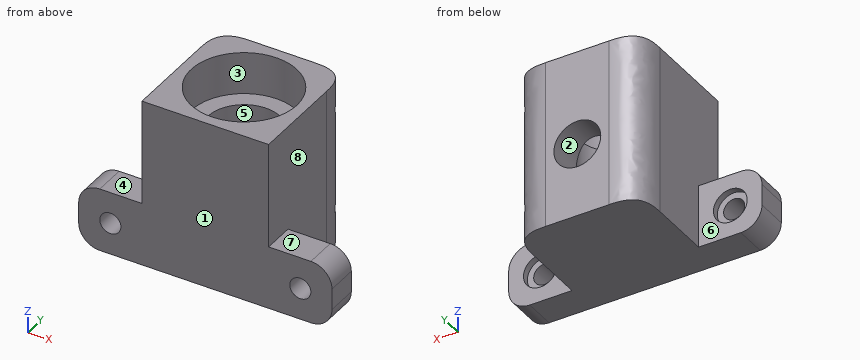
from build123d import *

# Parameters (mm, degrees)
BOSS_EXTRUDE1_DEPTH      = 35
BOSS_EXTRUDE1_DEPTH_BACK = 5
SKETCH1_W                = 30
SKETCH1_H                = 30
FILLET1_SIZE             = 7.5
SKETCH2_R                = 8.5
CUT_EXTRUDE1_DEPTH       = 60
SKETCH3_W                = 15
SKETCH3_H                = 7.5
BOSS_EXTRUDE2_DEPTH      = 15
SKETCH5_W                = 15
SKETCH5_H                = 7.5
BOSS_EXTRUDE4_DEPTH      = 15
SKETCH11_R               = 12.5
CUT_EXTRUDE3_DEPTH       = 10
FILLET8_R                = 5
SKETCH15_R               = 4
CUT_EXTRUDE5_DEPTH       = 1.5
SKETCH19_R               = 5.55625
CUT_EXTRUDE10_DEPTH      = 11.5
SKETCH21_R               = 2.5
CUT_EXTRUDE11_DEPTH      = 11.5


with BuildPart() as part:
    # Sketch1 → Boss-Extrude1 (new, two sides: drawn at the far end of the back side and taken through both)
    with BuildSketch(Plane.XY.offset(-BOSS_EXTRUDE1_DEPTH_BACK)):
        Rectangle(SKETCH1_W, SKETCH1_H)
    extrude(amount=BOSS_EXTRUDE1_DEPTH + BOSS_EXTRUDE1_DEPTH_BACK)

    # Fillet1
    # a fillet whose section is not a circle: 7.5 mm, written as the material it takes off along each edge
    with BuildSketch(Plane(origin=(-15, 15, 53.75), x_dir=(1, 0, 0), z_dir=(0, 0, -1))) as fillet1_piece_1:
        with BuildLine():
            add(Edge.make_bspline([(FILLET1_SIZE, 0), (FILLET1_SIZE * 0.831801948466, 0), (FILLET1_SIZE * 0.663603896932, 0), (FILLET1_SIZE * 0.292893218813, FILLET1_SIZE * 0.0716919198361), (FILLET1_SIZE * 0.0716919198361, FILLET1_SIZE * 0.292893218813), (0, FILLET1_SIZE * 0.663603896932), (0, FILLET1_SIZE * 0.831801948466), (0, FILLET1_SIZE)], knots=[0, 0, 0, 0, 0, 0, 0.5, 0.5, 1, 1, 1, 1, 1, 1], degree=5))
            Line((0, FILLET1_SIZE), (0, 0))
            Line((0, 0), (FILLET1_SIZE, 0))
        make_face()
    extrude(amount=77.5, mode=Mode.SUBTRACT)
    with BuildSketch(Plane(origin=(15, 15, -23.75), x_dir=(0, -1, 0), z_dir=(0, 0, 1))) as fillet1_piece_2:
        with BuildLine():
            add(Edge.make_bspline([(FILLET1_SIZE, 0), (FILLET1_SIZE * 0.831801948466, 0), (FILLET1_SIZE * 0.663603896932, 0), (FILLET1_SIZE * 0.292893218813, -FILLET1_SIZE * 0.0716919198361), (FILLET1_SIZE * 0.0716919198361, -FILLET1_SIZE * 0.292893218813), (0, -FILLET1_SIZE * 0.663603896932), (0, -FILLET1_SIZE * 0.831801948466), (0, -FILLET1_SIZE)], knots=[0, 0, 0, 0, 0, 0, 0.5, 0.5, 1, 1, 1, 1, 1, 1], degree=5))
            Line((0, -FILLET1_SIZE), (0, 0))
            Line((0, 0), (FILLET1_SIZE, 0))
        make_face()
    extrude(amount=77.5, mode=Mode.SUBTRACT)

    # Sketch2 → Cut-Extrude1 (cut)
    with BuildSketch(Plane.XY):
        with Locations(Location((0, 0, 0), (0, 0, 180))):
            Circle(SKETCH2_R)
    extrude(amount=CUT_EXTRUDE1_DEPTH, mode=Mode.SUBTRACT)

    # Sketch3 → Boss-Extrude2 (add)
    with BuildSketch(Plane(origin=(15, 0, 0), x_dir=(0, 0, -1), z_dir=(1, 0, 0))):
        with Locations((-2.5, -11.25)):
            Rectangle(SKETCH3_W, SKETCH3_H)
    extrude(amount=BOSS_EXTRUDE2_DEPTH)

    # Sketch5 → Boss-Extrude4 (add)
    with BuildSketch(Plane.ZY.offset(15)):
        with Locations((2.5, -11.25)):
            Rectangle(SKETCH5_W, SKETCH5_H)
    extrude(amount=BOSS_EXTRUDE4_DEPTH)

    # Sketch11 → Cut-Extrude3 (cut)
    with BuildSketch(Plane.XY.offset(35)):
        Circle(SKETCH11_R)
    extrude(amount=-CUT_EXTRUDE3_DEPTH, mode=Mode.SUBTRACT)

    # Fillet8
    fillet8_edges = [part.edges().sort_by_distance(p)[0] for p in [
        (30, -11.25, -5),
        (30, -11.25, 10),
        (-30, -11.25, -5),
        (-30, -11.25, 10),
    ]]
    fillet(fillet8_edges, radius=FILLET8_R)

    # Sketch15 → Cut-Extrude5 (cut)
    with BuildSketch(Plane(origin=(0, -7.5, 0), x_dir=(1, 0, 0), z_dir=(0, 1, 0))):
        with Locations(Location((22.5, -2.5, 0), (0, 0, 270))):
            Circle(SKETCH15_R)
        with Locations(Location((-22.5, -2.5, 0), (0, 0, 270))):
            Circle(SKETCH15_R)
    extrude(amount=-CUT_EXTRUDE5_DEPTH, mode=Mode.SUBTRACT)

    # Sketch19 → Cut-Extrude10 (cut)
    with BuildSketch(Plane(origin=(0, 15, 0), x_dir=(1, 0, 0), z_dir=(0, 1, 0))):
        with Locations(Location((0, -12.5, 0), (0, 0, 180))):
            Circle(SKETCH19_R)
    extrude(amount=-CUT_EXTRUDE10_DEPTH, mode=Mode.SUBTRACT)

    # Sketch21 → Cut-Extrude11 (cut)
    with BuildSketch(Plane(origin=(0, -9, 0), x_dir=(1, 0, 0), z_dir=(0, 1, 0))):
        with Locations(Location((-22.5, -2.5, 0), (0, 0, 270))):
            Circle(SKETCH21_R)
        with Locations(Location((22.5, -2.5, 0), (0, 0, 270))):
            Circle(SKETCH21_R)
    extrude(amount=-CUT_EXTRUDE11_DEPTH, mode=Mode.SUBTRACT)


solid = part.part
For this review, take the finished solid that the model builds, in its own axes (mm). Face numbers are marked on the shaded views. A direction names the side the tool comes from. Round coordinates to 2 decimals unless told otherwise and drop trailing zeros. Loops run counter-clockwise (first coordinate to the right, second up) from the corner with the lowest first, then second, coordinate; pieces in that order, holes last. Notation, with made-up numbers: (-32, 2.5) - (-23, 2.5) arc R26 cw to (-23, 32.5) - close; hole circle Ø1 at (-11.5, 65). An arc over 180 degrees is marked (long way). Answer as CSV lines item,"result".
(1) Tool access review of the marked faces 4, 5, 6, 7 and 8: name each direction out of +Z, -Z, +X, -X, +Y, -Y from which nothing blocks a thin tool from reaching the whole face with its end or side.
Checked values:
face 4,"+Z, -X, +Y, -Y"
face 5,"+Z"
face 6,"+Z, -Z, -X, +Y"
face 7,"+Z, +X, +Y, -Y"
face 8,"+Z, +X, +Y"
(2) Mouldability with a two-part tool opening along Y and no side actions: class the marked faces 1, 2 and 3 as +Y half, -Y half, draft (parallel to the pull), parting line (faces both ways), or undercut.
Checked values:
face 1,"-Y half"
face 2,"draft"
face 3,"undercut"
(3) Wall thickness on line 1 (X direction, y = -10.95, z = 2.5); line 2 (X direction, y = -0.5, z = 19.5); line 3 (Y direction, x = 0, z = 31.5): over which ranges is each line inside the solid? List them lowest first.
Checked values:
line 1,"x = -30 to -25, -20 to 20, 25 to 30"
line 2,"x = -15 to -8.49, 8.49 to 15"
line 3,"y = -15 to -12.5, 12.5 to 15"
(4) Consider section D-D on y = 0. Give the boundary of the cut face in (x, z), then the cut area to 3 significant figures.
Checked values:
outline,"(-15, -5) - (15, -5) - (15, 35) - (12.5, 35) - (12.5, 25) - (8.5, 25) - (8.5, 0) - (-8.5, 0) - (-8.5, 25) - (-12.5, 25) - (-12.5, 35) - (-15, 35) - close"
area,"525 mm2"
(5) Insertion check: P1, Ø13.5, axis at x = 2.5, y = -2.5, coming from the +Z side; P2, Ø7, axis at y = -7.5, z = 9, coming from the +X side; P3, Ø8, axis at y = -8.5, z = 15.5, coming from the -X side; P4, Ø2, axis at x = -17.5, z = 28.5, coming from the +Y side. Each pin has a flat end and moves straight along its axis. Give the tip position at first contact, or say it passes through.
Checked values:
P1,"stops at z = 25"
P2,"stops at x = 29.97"
P3,"stops at x = -15"
P4,"passes through"
(6) Consider section A-A on y = -10. Give the boundary of the cut face in (x, z).
Checked values:
outline,"(-30, 0) arc R5 ccw to (-25, -5) - (25, -5) arc R5 ccw to (30, 0) - (30, 5) arc R5 ccw to (25, 10) - (15, 10) - (15, 35) - (7.5, 35) - (7.5, 25) - (-7.5, 25) - (-7.5, 35) - (-15, 35) - (-15, 10) - (-25, 10) arc R5 ccw to (-30, 5) - close; hole circle Ø5 at (-22.5, 2.5); hole circle Ø5 at (22.5, 2.5)"
(7) Consider section B-B on x = 0. Give the boundary of the cut face in (y, z), then the cut area to 3 significant figures.
Checked values:
outline,"(-15, -5) - (15, -5) - (15, 6.94) - (8.5, 6.94) - (8.5, 0) - (-8.5, 0) - (-8.5, 25) - (-12.5, 25) - (-12.5, 35) - (-15, 35) - close; (8.5, 18.06) - (15, 18.06) - (15, 35) - (12.5, 35) - (12.5, 25) - (8.5, 25) - close"
area,"453 mm2"
(8) Consider section C-C on z = 2.5. Give the number of separate pieces and of enclosed holes in the cut face, then the cut area to 3 significant figures.
Checked values:
separate pieces,"3"
enclosed holes,"1"
area,"799 mm2"
